```python
from build123d import *

# Parameters (mm, degrees)
SKETCH_1_W          = 20
SKETCH_1_H          = 10
SKETCH_1_W_2        = 18
SKETCH_1_H_2        = 8
EXTRUDE_1_DEPTH     = 210
SKETCH_2_R          = 1.55
CUT_EXTRUDE_1_DEPTH = 212.187120819
SKETCH_3_R          = 1.55
CUT_EXTRUDE_2_DEPTH = 212.187120819


with BuildPart() as part:
    # 草图1 → 凸台-拉伸1 (new body)
    with BuildSketch(Plane.XY):
        with Locations((10, 5)):
            Rectangle(SKETCH_1_W, SKETCH_1_H)
        with Locations((10, 5)):
            Rectangle(SKETCH_1_W_2, SKETCH_1_H_2, mode=Mode.SUBTRACT)
    extrude(amount=EXTRUDE_1_DEPTH)

    # 草图2 → 切除-拉伸1 (cut, through all)
    with BuildSketch(Plane.XZ):
        with Locations(Location((5, 5, 0), (0, 0, 270))):
            Circle(SKETCH_2_R)
        with Locations(Location((15, 5, 0), (0, 0, 270))):
            Circle(SKETCH_2_R)
        with Locations(Location((15, 15, 0), (0, 0, 270))):
            Circle(SKETCH_2_R)
        with Locations(Location((5, 15, 0), (0, 0, 270))):
            Circle(SKETCH_2_R)
    extrude(amount=-CUT_EXTRUDE_1_DEPTH, mode=Mode.SUBTRACT)

    # 草图3 → 切除-拉伸2 (cut, through all)
    with BuildSketch(Plane.XZ):
        with Locations(Location((10, 200, 0), (0, 0, 270))):
            Circle(SKETCH_3_R)
        with Locations(Location((10, 185, 0), (0, 0, 270))):
            Circle(SKETCH_3_R)
        with Locations(Location((10, 170, 0), (0, 0, 270))):
            Circle(SKETCH_3_R)
        with Locations(Location((10, 155, 0), (0, 0, 270))):
            Circle(SKETCH_3_R)
        with Locations(Location((10, 140, 0), (0, 0, 270))):
            Circle(SKETCH_3_R)
        with Locations(Location((10, 125, 0), (0, 0, 270))):
            Circle(SKETCH_3_R)
        with Locations(Location((10, 110, 0), (0, 0, 270))):
            Circle(SKETCH_3_R)
    extrude(amount=-CUT_EXTRUDE_2_DEPTH, mode=Mode.SUBTRACT)


solid = part.part
```
Check sheet for the modelled part. Datum: model origin and axes. Units: mm. A direction names the side the tool comes from. Round coordinates to 2 decimals unless told otherwise and drop trailing zeros. Loops run counter-clockwise (first coordinate to the right, second up) from the corner with the lowest first, then second, coordinate; pieces in that order, holes last. Notation, with made-up numbers: (77, 13.5) - (81, 13.5) arc R20 cw to (81, 42.5) - close; hole circle Ø7 at (2, -17). An arc over 180 degrees is marked (long way). Write item = value, one per line. Start each with the question number.
Q1. Thickness scan on L1, parallel to X at y = 9.3, z = 15; L2, parallel to Y at x = 10.25, z = 115; L3, parallel to X at y = 0.7, z = 185. Record the ranges inside material, lowest first.
Q2. Section check A-A (y = 7.5). Record the boundary of the cut face in (x, z), plus the area to 3 significant figures.
Q3. Section check B-B (z = 58.5). Record the boundary of the cut face in (x, y).
Q4. Access from +Z, -Z, +X, -X, +Y, -Y to the whole of each face (thin tool, end or side, straight path). Record for faces 1 (the face through (10, 9, 104)), 2 (the face through (10, 10, 104)).
Q5. Release check for a two-part mould opening along X. For faces 3 (the face through (10, 0.6, 210)), 4 (the face through (1, 5, 104)), 5 (the face through (0, 5, 104)) record: pulls with the +X half, pulls with the -X half, needs draft (parallel to the pull), parting line crosses it, or undercut.
Derived:
q1.L1 = 0 to 3.45, 6.55 to 13.45, 16.55 to 20
q1.L2 = 0 to 1, 9 to 10
q1.L3 = 0 to 8.45, 11.55 to 20
q2.outline = (0, 0) - (1, 0) - (1, 210) - (0, 210) - close; (19, 0) - (20, 0) - (20, 210) - (19, 210) - close
q2.area = 420 mm^2
q3.outline = (0, 0) - (20, 0) - (20, 10) - (0, 10) - close; hole (1, 1) - (19, 1) - (19, 9) - (1, 9) - close
q4.face_1 = +Z, -Z
q4.face_2 = +Z, -Z, +X, -X, +Y
q5.face_3 = needs draft
q5.face_4 = undercut
q5.face_5 = pulls with the -X half
